CAD build for the part. Positions are in the model's coordinates, mm. Face numbers are marked on the shaded views. Round coordinates to 2 decimals unless told otherwise and drop trailing zeros. Loops run counter-clockwise (first coordinate to the right, second up) from the corner with the lowest first, then second, coordinate; pieces in that order, holes last. Notation, with made-up numbers: (-23, 64.5) - (32, 64.5) arc R26 cw to (32, 80.5) - close; hole circle Ø4 at (-36, -38). An arc over 180 degrees is marked (long way). Use one line per item in the form item = value.
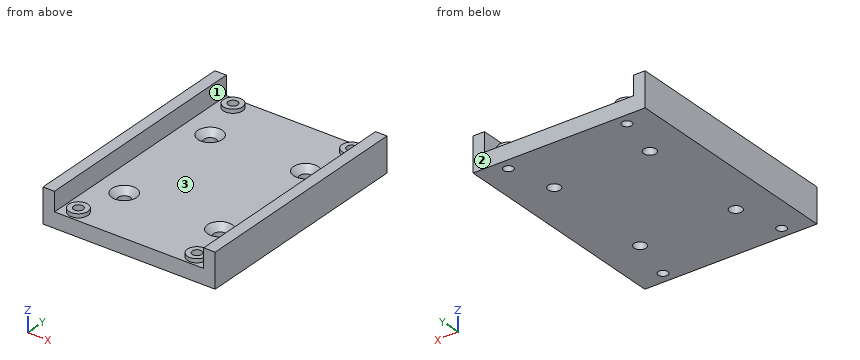
Autodesk Inventor part; units mm, degrees
ref_plane "YZ Plane" through (0, 0, 0) normal (1, 0, 0) x (0, 1, 0)
ref_plane "XZ Plane" through (0, 0, 0) normal (0, 1, 0) x (-1, 0, 0)
ref_plane "XY Plane" through (0, 0, 0) normal (0, 0, 1) x (1, 0, 0)
sketch "스케치1" plane through (0, 0, 0) normal (0, 0, 1) x (1, 0, 0)
  line L0 (-22.5, 30) -> (22.5, 30)
  line L1 (22.5, 30) -> (22.5, -30)
  line L2 (22.5, -30) -> (-22.5, -30)
  line L3 (-22.5, -30) -> (-22.5, 30)
  point P0 (0, 0)
  dimension "d0" = 45
  dimension "d1" = 60
  dimension "d2" = 30
  dimension "d3" = 22.5
extrude "돌출1" add sketch "스케치1" along normal blind 4
sketch "스케치2" plane through (0, 0, 4) normal (0, 0, 1) x (1, 0, 0)
  line L0 (-15.5, 27) -> (15.5, 27)
  line L1 (15.5, 27) -> (15.5, -27)
  line L2 (15.5, -27) -> (-15.5, -27)
  line L3 (-15.5, -27) -> (-15.5, 27)
  circle A0 centre (-15.5, 27) radius 1.25
  circle A1 centre (15.5, 27) radius 1.25
  circle A2 centre (-15.5, -27) radius 1.25
  circle A3 centre (15.5, -27) radius 1.25
  point P0 (0, 0)
  dimension "d6" = 31
  dimension "d7" = 54
  dimension "d8" = 15.5
  dimension "d9" = 27
  dimension "d10" = 2.5
  dimension "d11" = 2.5
  dimension "d12" = 2.5
  dimension "d13" = 2.5
extrude "돌출2" cut sketch "스케치2" against normal up to surface (4 mm away) contours L3 A0 L0 | L0 A0 L3 | A1 L1 L0 | L0 L1 A1 | A2 L2 L3 | L3 L2 A2 | A3 L2 L1 | L1 L2 A3
sketch "스케치3" plane through (0, 0, 4) normal (0, 0, 1) x (1, 0, 0)
  line L0 (-22.5, 30) -> (-22.5, -30)
  line L1 (-22.5, -30) -> (22.5, -30)
  line L2 (-22.5, 30) -> (-19.5, 30)
  line L3 (-19.5, 30) -> (-19.5, -30)
  line L4 (-19.5, -30) -> (-22.5, -30)
  line L5 (-22.5, -30) -> (-22.5, 30)
  line L6 (22.5, 30) -> (-22.5, 30)
  line L7 (22.5, 30) -> (19.5, 30)
  line L8 (19.5, 30) -> (19.5, -30)
  line L9 (19.5, -30) -> (22.5, -30)
  line L10 (22.5, -30) -> (22.5, 30)
  point P0 (0, 0)
  dimension "d16" = 3
  dimension "d17" = 3
extrude "돌출3" add sketch "스케치3" along normal blind 5 contours L2 L3 L1 L0 | L6 L10 L1 L8
sketch "스케치4" plane through (0, 0, 4) normal (0, 0, 1) x (1, 0, 0)
  circle A0 centre (-15.5, 27) radius 1.25
  circle A1 centre (15.5, 27) radius 1.25
  circle A2 centre (15.5, -27) radius 1.25
  circle A3 centre (-15.5, -27) radius 1.25
  circle A4 centre (-15.5, 27) radius 2.5
  circle A5 centre (-15.5, 27) radius 1.25
  circle A6 centre (15.5, 27) radius 2.5
  circle A7 centre (15.5, 27) radius 1.25
  circle A8 centre (15.5, -27) radius 2.5
  circle A9 centre (15.5, -27) radius 1.25
  circle A10 centre (-15.5, -27) radius 2.5
  circle A11 centre (-15.5, -27) radius 1.25
  point P0 (0, 0)
  dimension "d20" = 5
  dimension "d21" = 2.5
  dimension "d22" = 5
  dimension "d23" = 2.5
  dimension "d24" = 5
  dimension "d25" = 2.5
  dimension "d26" = 5
  dimension "d27" = 2.5
extrude "돌출4" add sketch "스케치4" along normal blind 1
sketch "스케치5" plane through (0, 0, 4) normal (0, 0, 1) x (1, 0, 0)
  line L0 (-12.5, 15) -> (12.5, 15)
  line L1 (12.5, 15) -> (12.5, -15)
  line L2 (12.5, -15) -> (-12.5, -15)
  line L3 (-12.5, -15) -> (-12.5, 15)
  circle A0 centre (-12.5, 15) radius 1.6
  circle A1 centre (12.5, 15) radius 1.6
  circle A2 centre (-12.5, -15) radius 1.6
  circle A3 centre (12.5, -15) radius 1.6
  point P0 (0, 0)
  dimension "d30" = 25
  dimension "d31" = 30
  dimension "d32" = 15
  dimension "d33" = 12.5
  dimension "d34" = 3.2
  dimension "d35" = 3.2
  dimension "d36" = 3.2
  dimension "d37" = 3.2
extrude "돌출5" cut sketch "스케치5" against normal up to surface (4 mm away) contours L3 A0 L0 | L0 A0 L3 | A1 L1 L0 | L0 L1 A1 | A2 L2 L3 | L3 L2 A2 | A3 L2 L1 | L1 L2 A3
chamfer "모따기1" distance 1.6 angle 45 4 edges at (10.9, -15, 4) (-14.1, -15, 4) (10.9, 15, 4) (-14.1, 15, 4)
properties part number "회로프레임" material "LCP 플라스틱"
1) Drill centre lines: probe 1 along Y at (x, z) = (15.5, 1.8); probe 2 along X at (y, z) = (15, 1.9); probe 3 along Y at (x, z) = (12.5, 0.95). Where is each one in solid material? Low to high.
Report:
probe_1 = -30 to -28.25, -25.75 to 25.75, 28.25 to 30
probe_2 = -22.5 to -14.1, -10.9 to 10.9, 14.1 to 22.5
probe_3 = -30 to -16.6, -13.4 to 13.4, 16.6 to 30
2) Slice it at D-D (x = 8). Write the cut outline in (y, z), plus the area to 3 significant figures.
Report:
outline = (-30, 0) - (30, 0) - (30, 4) - (-30, 4) - close
area = 240 mm^2
3) Slice it at A-A (y = 15). Write the cut outline in (x, z).
Report:
outline = (-22.5, 0) - (-14.1, 0) - (-14.1, 2.4) - (-15.7, 4) - (-19.5, 4) - (-19.5, 9) - (-22.5, 9) - close; (-10.9, 0) - (10.9, 0) - (10.9, 2.4) - (9.3, 4) - (-9.3, 4) - (-10.9, 2.4) - close; (14.1, 0) - (22.5, 0) - (22.5, 9) - (19.5, 9) - (19.5, 4) - (15.7, 4) - (14.1, 2.4) - close
4) Slice it at C-C (y = -5.5). Write the cut outline in (x, z), plus the area to 3 significant figures.
Report:
outline = (-22.5, 0) - (22.5, 0) - (22.5, 9) - (19.5, 9) - (19.5, 4) - (-19.5, 4) - (-19.5, 9) - (-22.5, 9) - close
area = 210 mm^2
5) Slice it at B-B (z = 1.5). State how many separate pieces and enclosed holes the cut face has, plus the area to 3 significant figures.
Report:
separate_pieces = 1
enclosed_holes = 8
area = 2,650 mm^2
6) Flat gauge pins, fed straight in: pin 1 (1.5 mm diameter, centred on x = 15.5, y = -26, fed in from +Z); pin 2 (3 mm diameter, centred on x = -14, y = -4, fed in from +Z); pin 3 (1.5 mm diameter, centred on x = 13.5, z = 5, fed in from +Y). Where does each tip first touch, or does it go through?
Report:
pin_1 = 5
pin_2 = 4
pin_3 = 29.17
7) Two-plate mould, pull along Y, no slides. Class the marked faces 1, 2 and 3: +Y half, -Y half, draft (parallel to the pull), parting line (faces both ways), or undercut.
Report:
face_1 = draft
face_2 = +Y half
face_3 = undercut
